Source: three-view drawing plus pictorial views. Frame: mm from the lowest corner of the part. A direction names the side the tool comes from. Round coordinates to 2 decimals unless told otherwise and drop trailing zeros. Loops run counter-clockwise (first coordinate to the right, second up) from the corner with the lowest first, then second, coordinate; pieces in that order, holes last. Notation, with made-up numbers: (-3.75, 76.25) -> (4.25, 76.25) arc R24 ccw to (4.25, 103.25) -> close; hole circle Ø6 at (24.5, 11). An arc over 180 degrees is marked (long way). One line per question, with ' | ' between items. Start each with the question number.
Q1. Contact query for flat-ended pins moving along their axis: P1, Ø2, axis at y = 8.5, z = 7.5, coming from the -X side; P2, Ø2, axis at x = 7.5, z = 11, coming from the +Y side; P3, Ø2, axis at x = 14, y = 2, coming from the +Z side; P4, Ø4, axis at x = 2, z = 15, coming from the +Y side. Output: stop coordinate, or through.
Q2. Mould query, pull axis Z, two halves, no side actions, for the marked faces 6, 7 and 8. Classes: pulls with the +Z half, pulls with the -Z half, needs draft (parallel to the pull), parting line crosses it, or undercut.
Q3. Cut plane C-C on z = 12.75. Return loops of the section in (x, y).
Q4. Access query for the marked faces 1, 2, 3, 4 and 5. Directions: +Z, -Z, +X, -X, +Y, -Y. A direction counts if a zero-diameter tool reaches every point of the face in a straight line with its end or side. Return the directions, or none.
Q5. Cut plane D-D on z = 18. Return loops of the section in (x, y).
Q6. Cut plane A-A on y = 7.5. Return loops of the section in (x, z).
Q7. Material intervals for L1, parallel to X at y = 8, z = 9.5; L2, parallel to Z at x = 4.95, y = 7.5; L3, parallel to Y at x = 3.5, z = 12.5, sorted ascending.
Q8. Cut plane B-B on x = 4.5. Return loops of the section in (y, z).
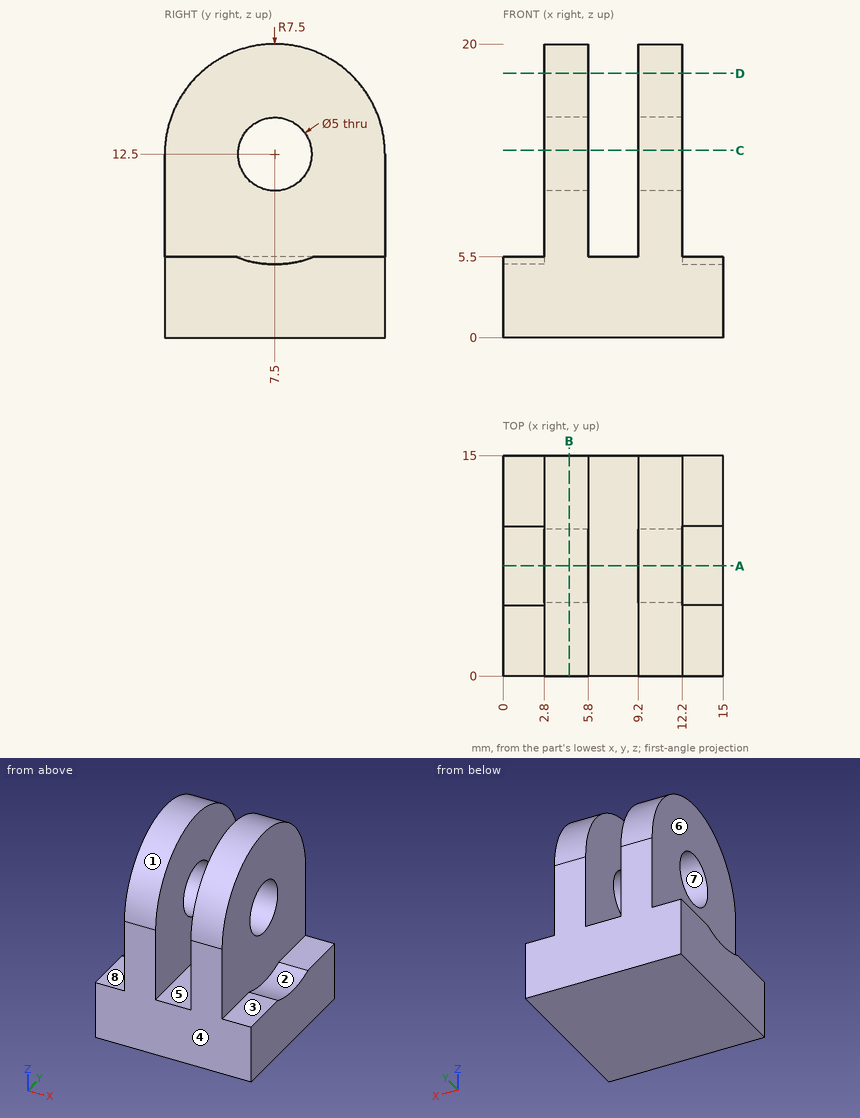
Results:
1) P1: x = 2.8 | P2: through | P3: z = 5.5 | P4: y = 14.97
2) face 6: needs draft | face 7: undercut | face 8: pulls with the +Z half
3) outline: (2.8, 0) -> (5.8, 0) -> (5.8, 5.01) -> (2.8, 5.01) -> close; (2.8, 9.99) -> (5.8, 9.99) -> (5.8, 15) -> (2.8, 15) -> close; (9.2, 0) -> (12.2, 0) -> (12.2, 5.01) -> (9.2, 5.01) -> close; (9.2, 9.99) -> (12.2, 9.99) -> (12.2, 15) -> (9.2, 15) -> close
4) face 1: +Z, +X, -X | face 2: +Z, +X | face 3: +Z, +X, +Y, -Y | face 4: +Z, -Z, +X, -X, -Y | face 5: +Z, +Y, -Y
5) outline: (2.8, 2.4) -> (5.8, 2.4) -> (5.8, 12.6) -> (2.8, 12.6) -> close; (9.2, 2.4) -> (12.2, 2.4) -> (12.2, 12.6) -> (9.2, 12.6) -> close
6) outline: (0, 0) -> (15, 0) -> (15, 5) -> (12.2, 5) -> (12.2, 10) -> (9.2, 10) -> (9.2, 5.5) -> (5.8, 5.5) -> (5.8, 10) -> (2.8, 10) -> (2.8, 5) -> (0, 5) -> close; (2.8, 15) -> (5.8, 15) -> (5.8, 20) -> (2.8, 20) -> close; (9.2, 15) -> (12.2, 15) -> (12.2, 20) -> (9.2, 20) -> close
7) L1: 2.8 to 5.8, 9.2 to 12.2 | L2: 0 to 10, 15 to 20 | L3: 0 to 5, 10 to 15
8) outline: (0, 0) -> (15, 0) -> (15, 12.5) arc R7.5 ccw to (0, 12.5) -> close; hole circle Ø5 at (7.5, 12.5)
